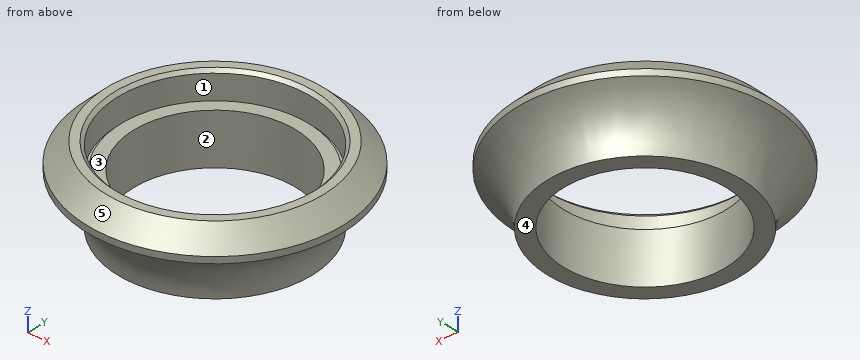
```python
from build123d import *

# Parameters (mm, degrees)
F2_SIZE = 0.5


with BuildPart() as f1:
    # F0 (on Front) → F1 (revolve)
    with BuildSketch(Plane.XZ):
        with BuildLine():
            Line((12.7, 8), (12.7, 0))
            Line((12.7, 0), (15.2, 0))
            ThreePointArc((15.2, 0), (16.492064, 4.664762), (20, 8))
            Line((20, 8), (20, 9))
            Line((20, 9), (17, 12))
            Line((17, 12), (15.2, 12))
            Line((15.2, 12), (15.2, 7.5))
            Line((15.2, 7.5), (14.7, 7.5))
            Line((14.7, 7.5), (14.7, 8))
            Line((14.7, 8), (12.7, 8))
        make_face()
    revolve(axis=Axis((0, 0, 6), (0, 0, 1)))

    # F2
    f2_edges = [f1.edges().sort_by_distance(p)[0] for p in [
        (-15.2, 0, 12),
    ]]
    chamfer(f2_edges, length=F2_SIZE)


solid = f1.part
```
Work out the finished part from the listing and answer in its coordinate system (mm). Face numbers are marked on the shaded views. A direction names the side the tool comes from. Round coordinates to 2 decimals unless told otherwise and drop trailing zeros. Loops run counter-clockwise (first coordinate to the right, second up) from the corner with the lowest first, then second, coordinate; pieces in that order, holes last.
(1) The mould has two halves that part along X. Classify the marked faces 3, 4 and 5: pulls with the +X half, pulls with the -X half, needs draft (parallel to the pull), parting line crosses it, or undercut.
Computed values:
face 3: undercut
face 4: needs draft
face 5: parting line crosses it
(2) The part is cut by section A-A, the plane y = 0. Give the vertices of the cut face in (x, z).
Computed values:
outline: (-20, 8) arc R9.07 cw to (-15.2, 0) - (-12.7, 0) - (-12.7, 8) - (-14.7, 8) - (-14.7, 7.5) - (-15.2, 7.5) - (-15.2, 11.5) - (-15.7, 12) - (-17, 12) - (-20, 9) - close; (12.7, 0) - (15.2, 0) arc R9.07 cw to (20, 8) - (20, 9) - (17, 12) - (15.7, 12) - (15.2, 11.5) - (15.2, 7.5) - (14.7, 7.5) - (14.7, 8) - (12.7, 8) - close
(3) The part is cut by section C-C, the plane z = 10.75. Give the vertices of the cut face in (x, y).
Computed values:
outline: circle Ø36.5 at (0, 0); hole circle Ø30.4 at (0, 0)
(4) Each of these flat-tipped pins is pushed along its axis until it touches: P1, Ø1, axis at x = -8.5, y = 14, coming from the -Z side; P2, Ø15, axis at x = 0, y = 0, coming from the +Z side; P3, Ø1, axis at x = 4, z = 2.5, coming from the +Y side; P4, Ø4, axis at y = 9.5, z = 3, coming from the +X side. Where does it stop, or does it pass through?
Computed values:
P1: stops at z = 3.44
P2: passes through
P3: stops at y = 15.23
P4: stops at x = 14.21
(5) For the marked faces 1 and 2, determine the directions among +Z, -Z, +X, -X, +Y, -Y from which every point of the face is accessible in a straight line to the end or side of a thin tool.
Computed values:
face 1: +Z
face 2: +Z, -Z
(6) The part is cut by section D-D, the plane z = 3.25. Give the vertices of the cut face in (x, y), and give its area (3 significant figures).
Computed values:
outline: circle Ø31.61 at (0, 0); hole circle Ø25.4 at (0, 0)
area: 278 mm2
(7) Find the intervals of material crossed by L1, parallel to Y at x = 3, z = 7.75; L2, parallel to Z at x = -3.5, y = 14.5; L3, parallel to Z at x = -7.5, y = 12.5, in increasing order.
Computed values:
L1: y = -19.33 to -14.9, -14.39 to -12.34, 12.34 to 14.39, 14.9 to 19.33
L2: z = 0 to 7.5
L3: z = 0 to 8
